```python
from build123d import *

# Parameters (mm, degrees)
SKETCH1_W           = 100
SKETCH1_H           = 10
BOSS_EXTRUDE1_DEPTH = 20
SKETCH2_R           = 2.713153407
SKETCH2_R_2         = 2.694189889
SKETCH2_R_3         = 2.523769014
BOSS_EXTRUDE2_DEPTH = 8


with BuildPart() as part:
    # Sketch1 → Boss-Extrude1 (new body)
    with BuildSketch(Plane(origin=(0, 0, 0), x_dir=(1, 0, 0), z_dir=(0, 1, 0))):
        Rectangle(SKETCH1_W, SKETCH1_H)
    extrude(amount=BOSS_EXTRUDE1_DEPTH)

    # Sketch2 → Boss-Extrude2 (add)
    with BuildSketch(Plane(origin=(0, 20, 0), x_dir=(1, 0, 0), z_dir=(0, 1, 0))):
        with Locations(Location((-43.29861016, 0, 0), (0, 0, 270))):
            Circle(SKETCH2_R)
        with Locations(Location((-36.758074643, 0, 0), (0, 0, 270))):
            Circle(SKETCH2_R)
        with Locations(Location((-22.408108815, -0.328361024, 0), (0, 0, 270))):
            Circle(SKETCH2_R)
        with Locations(Location((-15.867573299, -0.328361024, 0), (0, 0, 270))):
            Circle(SKETCH2_R)
        with Locations(Location((17.140046294, -0.119001471, 0), (0, 0, 270))):
            Circle(SKETCH2_R_2)
        with Locations(Location((23.146948699, -0.119001471, 0), (0, 0, 270))):
            Circle(SKETCH2_R_2)
        with Locations(Location((38.761600382, -0.119001471, 0), (0, 0, 270))):
            Circle(SKETCH2_R_3)
        with Locations(Location((44.898381169, -0.119001471, 0), (0, 0, 270))):
            Circle(SKETCH2_R_3)
        with Locations(Location((-3.447043883, -0.524988506, 0), (0, 0, 270))):
            Circle(SKETCH2_R)
        with Locations(Location((3.093491634, -0.524988506, 0), (0, 0, 270))):
            Circle(SKETCH2_R)
    extrude(amount=BOSS_EXTRUDE2_DEPTH)


solid = part.part
```
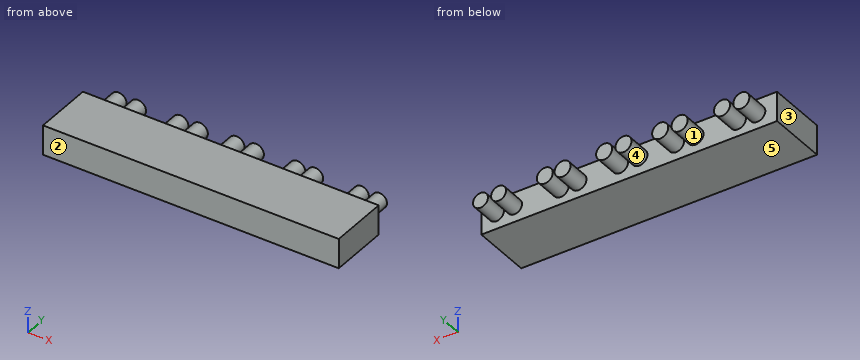
Geometry: final body of the model. Coordinates: model frame, mm. Face numbers are marked on the shaded views. A direction names the side the tool comes from. Coordinates: 2 decimals unless noted, no trailing zeros. Order: outer loops, then holes, each group sorted by start corner. A loop starts at its lowest first (then second) coordinate and runs counter-clockwise, first axis right, second up. Notation, with made-up numbers: (46.5, 25) - (65.5, 25) arc R22 cw to (65.5, 32) - close; hole circle Ø3 at (-6.75, 12.25). An arc over 180 degrees is marked (long way). Write each question's results on one line, items separated by ' | '.
(1) Mould query, pull axis X, two halves, no side actions, for the marked faces 3, 4 and 5. Classes: +X half, -X half, draft (parallel to the pull), parting line (faces both ways), or undercut.
Values found:
face 3: -X half | face 4: undercut | face 5: draft
(2) Section query C-C, the plane x = 9. Return the cut outline in (y, z).
Values found:
outline: (0, -5) - (20, -5) - (20, 5) - (0, 5) - close
(3) Section query A-A, the plane y = 26.25. Count the separate pieces of the cut face and the enclosed holes in it, plus the area to 3 significant figures.
Values found:
separate pieces: 10 | enclosed holes: 0 | area: 224 mm²
(4) First-contact query: pin 1 Ø1 at (x, z) = (12, -2.5) entering from -Y; pin 2 Ø4 at (x, z) = (9.5, 2) entering from +Y. Flat tips, straight axial feed; report the tip coordinate or a pass-through.
Values found:
pin 1: stops at y = 0 | pin 2: stops at y = 20
(5) Set-up query: the marked faces 1 and 2. Return all of +Z, -Z, +X, -X, +Y, -Y with unobstructed straight access to the full face (end or side cutting, diameter ignored); none if empty.
Values found:
face 1: +Y | face 2: +Z, -Z, +X, -X, -Y
(6) Section query B-B, the plane x = -24. Return the cut outline in (y, z).
Values found:
outline: (0, -5) - (20, -5) - (20, -1.87) - (28, -1.87) - (28, 2.53) - (20, 2.53) - (20, 5) - (0, 5) - close
(7) Line query: line 1 (Y direction, x = -35.5, z = -4.5); line 2 (Z direction, x = 17.5, y = 26). Output: solid intervals per line, ascending. Write a range as [from, to].
Values found:
line 1: y = [0, 20] | line 2: z = [-2.55, 2.79]
